Verification items for the finished model (mm, model axes). A direction names the side the tool comes from. Round coordinates to 2 decimals unless told otherwise and drop trailing zeros. Write each loop counter-clockwise with the first axis right and the second up, starting at its lowest first coordinate (ties: lowest second). Pieces come first, ordered by that corner, then holes. Notation, with made-up numbers: M 35.25,57 L 81.25,57 A7 ccw 81.25,69 Z; hole C 40.5,14.5 d4. An arc over 180 degrees is marked long. One line per question, with ' | ' between items.
from build123d import *

# Parameters (mm, degrees)
F1_DEPTH = 25.4
F3_DEPTH = 25.4
F5_DEPTH = 25.4


with BuildPart() as f1:
    # F0 (on Front) → F1 (new body)
    with BuildSketch(Plane.XZ):
        Polygon((0, 31.75), (0, 0), (57.15, 0), (44.45, 31.75), align=None)
    extrude(amount=F1_DEPTH)

    # F2 (on face) → F3 (join)
    with BuildSketch(Plane.XZ.offset(25.4)):
        Polygon((0, 31.75), (0, 0), (44.45, 0), (19.05, 31.75), align=None)
    extrude(amount=F3_DEPTH)

    # F4 (on face) → F5 (join)
    with BuildSketch(Plane(origin=(0, 0, 0), x_dir=(-1, 0, 0), z_dir=(0, 1, 0))):
        Polygon((-44.45, 0), (0, 0), (0, 31.75), (-22.225, 31.75), align=None)
    extrude(amount=F5_DEPTH)


solid = f1.part
1. Section check A-A, the plane z = 22.5. Record the cut outline in (x, y).
Results:
outline: M 0,-50.8 L 26.45,-50.8 L 26.45,-25.4 L 48.15,-25.4 L 48.15,0 L 28.7,0 L 28.7,25.4 L 0,25.4 Z
2. Tool access check on faces 1 (the face through (39, 0, 16)), 2 (the face through (0, -13, 16)), 3 (the face through (31.93, -37.92, 15.65)). Record the directions out of +Z, -Z, +X, -X, +Y, -Y that give a thin tool (end or side, any length) a straight path to the whole face; none if there is none.
Results:
face 1: +Z, +X, +Y | face 2: +Z, -Z, -X, +Y, -Y | face 3: +Z, +X, -Y
3. Section check D-D, the plane y = -46. Record the cut outline in (x, z).
Results:
outline: M 0,0 L 44.45,0 L 19.05,31.75 L 0,31.75 Z
4. Thickness scan on line 1 (Y direction, x = 26, z = 30); line 2 (Z direction, x = 42, y = 8); line 3 (X direction, y = 17.5, z = 9). Record the ranges inside material, lowest first.
Results:
line 1: y = -25.4 to 0 | line 2: z = 0 to 3.5 | line 3: x = 0 to 38.15
5. Section check C-C, the plane y = -22. Record the cut outline in (x, z).
Results:
outline: M 0,0 L 57.15,0 L 44.45,31.75 L 0,31.75 Z
6. Section check B-B, the plane x = 25. Record the cut outline in (y, z).
Results:
outline: M -50.8,0 L 25.4,0 L 25.4,27.79 L 0,27.79 L 0,31.75 L -25.4,31.75 L -25.4,24.31 L -50.8,24.31 Z
7. Go/stop test with flat-tipped pins: P1, Ø12, axis at x = 50.5, z = 27.5, coming from the +Y side; P2, Ø3, axis at y = 11.5, z = 28, coming from the +X side; P3, Ø10, axis at y = -3, z = 5, coming from the -X side; P4, Ø9.5, axis at x = 45.5, z = 12.5, coming from the -Y side. Record where each tip stops, or that it passes through.
Results:
P1: stops at y = 0 | P2: stops at x = 25.9 | P3: stops at x = 0 | P4: stops at y = -25.4
